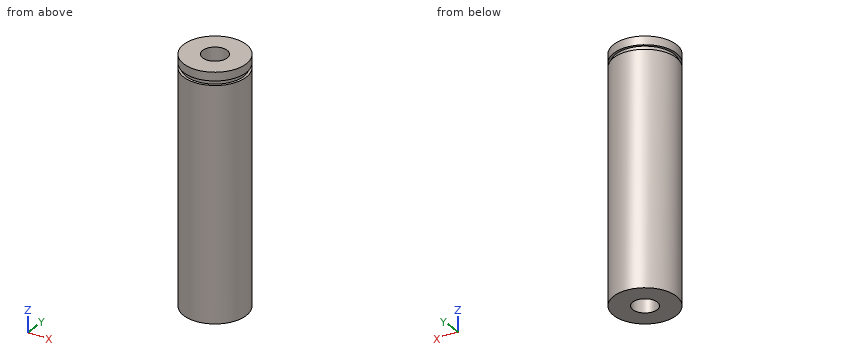
from build123d import *

# Parameters (mm, degrees)
SKETCH1_R           = 6.35
SKETCH1_R_2         = 2.4892
BOSS_EXTRUDE1_DEPTH = 24.6888
SKETCH2_W           = 0.889
SKETCH2_H           = 1.0033


with BuildPart() as part:
    # Sketch1 → Boss-Extrude1 (new, symmetric)
    with BuildSketch(Plane.XY):
        Circle(SKETCH1_R)
        Circle(SKETCH1_R_2, mode=Mode.SUBTRACT)
    extrude(amount=BOSS_EXTRUDE1_DEPTH, both=True)

    # Sketch2 → Cut-Revolve1 (revolve, cut)
    with BuildSketch(Plane(origin=(0, 0, 0), x_dir=(0, 0, -1), z_dir=(1, 0, 0)), mode=Mode.PRIVATE) as cut_revolve1_sk:
        with Locations((-22.5298, 6.35635)):
            Rectangle(SKETCH2_W, SKETCH2_H)
    revolve(cut_revolve1_sk.sketch.rotate(Axis((0, 0, 2.405637885), (0, 0, -1)), 90), axis=Axis((0, 0, 2.405637885), (0, 0, -1)), mode=Mode.SUBTRACT)


solid = part.part
Work out the finished part from the listing and answer in its coordinate system (mm). Give positions to 0.01 mm unless a question says otherwise; leave off trailing zeros. Order: outer loops, then holes, each group sorted by start corner. A loop starts at its lowest first (then second) coordinate and runs counter-clockwise, first axis right, second up. Notation, with made-up numbers: (20.25, -21) -> (32.25, -21) arc R12 ccw to (32.25, -15) -> close; hole circle Ø2 at (28.25, 31). An arc over 180 degrees is marked (long way). One line per item, written item: value.
Item 1: Find section A-A, the plane x = 0. Give the vertices of the cut face in (y, z).
Answer sheet:
outline: (-6.35, -24.69) -> (-2.49, -24.69) -> (-2.49, 24.69) -> (-6.35, 24.69) -> (-6.35, 22.97) -> (-5.85, 22.97) -> (-5.85, 22.09) -> (-6.35, 22.09) -> close; (2.49, -24.69) -> (6.35, -24.69) -> (6.35, 22.09) -> (5.85, 22.09) -> (5.85, 22.97) -> (6.35, 22.97) -> (6.35, 24.69) -> (2.49, 24.69) -> close
Item 2: Find section C-C, the plane z = -11. Give the vertices of the cut face in (x, y), plus the area to 3 significant figures.
Answer sheet:
outline: circle Ø12.7 at (0, 0); hole circle Ø4.98 at (0, 0)
area: 107 mm²
Item 3: Find section D-D, the plane y = 4. Give the vertices of the cut face in (x, z).
Answer sheet:
outline: (-4.93, -24.69) -> (4.93, -24.69) -> (4.93, 22.09) -> (4.28, 22.09) -> (4.28, 22.97) -> (4.93, 22.97) -> (4.93, 24.69) -> (-4.93, 24.69) -> (-4.93, 22.97) -> (-4.28, 22.97) -> (-4.28, 22.09) -> (-4.93, 22.09) -> close
Item 4: Straight lines are drawn through the part: probe 1 along Y at (x, z) = (0, 13.5); probe 2 along Y at (x, z) = (-1.25, -17); probe 3 along X at (y, z) = (0.25, -9.5). For each, find the intervals that lie inside material, in ascending order.
Answer sheet:
probe 1: -6.35 to -2.49, 2.49 to 6.35
probe 2: -6.23 to -2.15, 2.15 to 6.23
probe 3: -6.35 to -2.48, 2.48 to 6.35
Item 5: Flat-ended cylindrical pins translate along their axes: P1, Ø1, axis at x = 2.5, z = 5.5, coming from the +Y side; P2, Ø1, axis at y = -5, z = -18, coming from the -X side; P3, Ø4, axis at x = -4, z = 12, coming from the -Y side. Find the tip coordinate at first contact, or state that the pin passes through.
Answer sheet:
P1: y = 6.03
P2: x = -4.48
P3: y = -6.03
